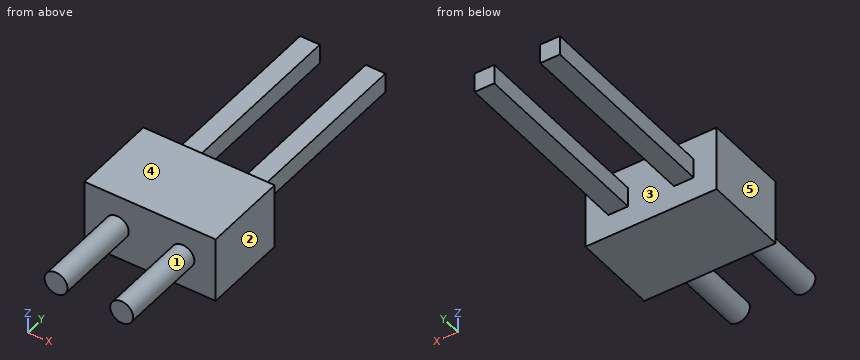
Autodesk Inventor part; units mm, degrees
ref_plane "YZ Plane (RIGHT)" through (0, 0, 0) normal (1, 0, 0) x (0, 1, 0)
ref_plane "XZ Plane (TOP)" through (0, 0, 0) normal (0, 1, 0) x (-1, 0, 0)
ref_plane "XY Plane (FRONT)" through (0, 0, 0) normal (0, 0, 1) x (1, 0, 0)
sketch "Sketch2" plane through (0, 0, 0) normal (0, 0, 1) x (1, 0, 0)
  line L0 (-1.778, 0) -> (1.778, 0) construction
  line L1 (0, 3.9624) -> (0, -0.6604) construction
  line L2 (-1.27, 3.302) -> (1.27, 3.302)
  line L3 (1.27, 3.302) -> (1.27, 0)
  line L4 (1.27, 0) -> (-1.27, 0)
  line L5 (-1.27, 0) -> (-1.27, 3.302)
  point P0 (0, 0)
  dimension "d0" = 2.54
  dimension "d1" = 3.302
extrude "Extrusion1" add sketch "Sketch2" along normal mid plane 2.54
sketch "Sketch3" plane through (-1.27, 0, 1.27) normal (0, -1, 0) x (1, 0, 0)
  circle A0 centre (1.27, -1.27) radius 0.4445
  line L0 (1.27, 0.508) -> (1.27, -3.048) construction
  line L1 (-0.508, -1.27) -> (3.048, -1.27) construction
  line L2 (0.889, -0.889) -> (1.651, -0.889)
  line L3 (1.651, -0.889) -> (1.651, -1.651)
  line L4 (1.651, -1.651) -> (0.889, -1.651)
  line L5 (0.889, -1.651) -> (0.889, -0.889)
  dimension "d4" = 0.762
  dimension "d5" = 0.889
extrude "Extrusion2" add sketch "Sketch3" against normal blind 10.795 contours L3 A0 L4 L5 L2 | A0 L2 L3 | L3 L4 A0 | A0 L5 L2 | L4 L5 A0
extrude "Extrusion3" add sketch "Sketch3" along normal blind 3.429 contours A0 L3 | L3 A0 L4 L5 L2 | L2 A0 | A0 L4 | L5 A0
pattern_linear "Rectangular Pattern1" count 2 spacing 2.54 along (1, 0, 0) of "Extrusion1", "Extrusion2", "Extrusion3"
properties part number "Jumper 2 Pin"
Can you work these out from the model? Positions are in its coordinate system, mm. Face numbers are marked on the shaded views. A direction names the side the tool comes from. Round coordinates to 2 decimals unless told otherwise and drop trailing zeros. Write each loop counter-clockwise with the first axis right and the second up, starting at its lowest first coordinate (ties: lowest second). Pieces come first, ordered by that corner, then holes. Notation, with made-up numbers: M 56,-32 L 90,-32 A16 cw 90,-17 Z; hole C 32.25,23 d6. An arc over 180 degrees is marked long. Use a Markdown table: item, result.
Item 1: We'd pull the mould along X, two halves only. Please class the marked faces 3, 4 and 5: released by +X, released by -X, zero draft, split by the parting line, or undercut.
Found:
| item | result |
|---|---|
| face 3 | undercut |
| face 4 | zero draft |
| face 5 | released by -X |
Item 2: Which directions (+Z, -Z, +X, -X, +Y, -Y) give clear straight access to the entire face, cutting with the end or side of a thin tool? Please do the marked faces 1 and 2.
Found:
| item | result |
|---|---|
| face 1 | -Y |
| face 2 | +Z, -Z, +X, +Y, -Y |
Item 3: For pin 1 Ø0.6 at (x, y) = (0, 7.5) entering from +Z; pin 2 Ø1 at (x, y) = (1, 6) entering from +Z; pin 3 Ø0.8 at (y, z) = (8, 0) entering from +X; pin 4 Ø0.6 at (x, y) = (0, 5.5) entering from -Z, each with a flat end and sliding along its axis, tell me the tip position at first contact or that it passes through.
Found:
| item | result |
|---|---|
| pin 1 | stops at z = 0.38 |
| pin 2 | passes through |
| pin 3 | stops at x = 2.92 |
| pin 4 | stops at z = -0.38 |
Item 4: I want a section at A-A (z = 0). List the corners of the cut face in (x, y) for me (1 decimal).
Found:
| item | result |
|---|---|
| outline | M -1.3,0 L -0.4,0 L -0.4,-3.4 L 0.4,-3.4 L 0.4,0 L 2.1,0 L 2.1,-3.4 L 3,-3.4 L 3,0 L 3.8,0 L 3.8,3.3 L 2.9,3.3 L 2.9,10.8 L 2.2,10.8 L 2.2,3.3 L 0.4,3.3 L 0.4,10.8 L -0.4,10.8 L -0.4,3.3 L -1.3,3.3 Z |
Item 5: If I drill on line 1 along X through (y, z) = (8, 0.3); line 2 along Y through (x, z) = (1.45, 0.5); line 3 along X through (y, z) = (-2.5, 0.3), over which ranges is the centre line in solid material (lowest first)? Write a range as [from, to].
Found:
| item | result |
|---|---|
| line 1 | x = [-0.38, 0.38], [2.16, 2.92] |
| line 2 | y = [0, 3.3] |
| line 3 | x = [-0.33, 0.33], [2.21, 2.87] |
Item 6: I want a section at D-D (x = 2.35). List the corners of the cut face in (y, z) for me (3 decimals), and give its area (3 significant figures).
Found:
| item | result |
|---|---|
| outline | M -3.429,-0.402 L 0,-0.402 L 0,-1.27 L 3.302,-1.27 L 3.302,-0.381 L 10.795,-0.381 L 10.795,0.381 L 3.302,0.381 L 3.302,1.27 L 0,1.27 L 0,0.402 L -3.429,0.402 Z |
| area | 16.9 mm2 |
Item 7: I want a section at B-B (x = 0). List the corners of the cut face in (y, z) for me (1 decimal), and give its area (3 significant figures).
Found:
| item | result |
|---|---|
| outline | M -3.4,-0.4 L 0,-0.4 L 0,-1.3 L 3.3,-1.3 L 3.3,-0.4 L 10.8,-0.4 L 10.8,0.4 L 3.3,0.4 L 3.3,1.3 L 0,1.3 L 0,0.4 L -3.4,0.4 Z |
| area | 17.1 mm2 |
Item 8: I want a section at C-C (y = -1.25). List the corners of the cut face in (x, z) for me.
Found:
| item | result |
|---|---|
| outline | C 0,0 d0.89; C 2.54,0 d0.89 |
